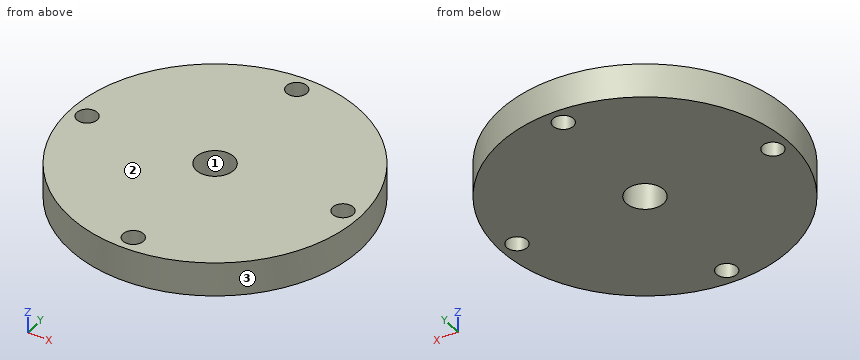
from build123d import *

# Parameters (mm, degrees)
ESQUISSE1_R        = 4.25
ESQUISSE1_R_2      = 0.3
ESQUISSE1_R_3      = 0.55
BOSS_EXTRU_1_DEPTH = 1


with BuildPart() as part:
    # Esquisse1 → Boss.-Extru.1 (new body)
    with BuildSketch(Plane.XY):
        Circle(ESQUISSE1_R)
        with Locations((0, 3.75)):
            Circle(ESQUISSE1_R_2, mode=Mode.SUBTRACT)
        Circle(ESQUISSE1_R_3, mode=Mode.SUBTRACT)
        with Locations((3.75, 0)):
            Circle(ESQUISSE1_R_2, mode=Mode.SUBTRACT)
        with Locations((0, -3.75)):
            Circle(ESQUISSE1_R_2, mode=Mode.SUBTRACT)
        with Locations((-3.75, 0)):
            Circle(ESQUISSE1_R_2, mode=Mode.SUBTRACT)
    extrude(amount=BOSS_EXTRU_1_DEPTH)


solid = part.part
For this review, take the finished solid that the model builds, in its own axes (mm). Face numbers are marked on the shaded views. Round coordinates to 2 decimals unless told otherwise and drop trailing zeros. Order: outer loops, then holes, each group sorted by start corner. A loop starts at its lowest first (then second) coordinate and runs counter-clockwise, first axis right, second up. Notation, with made-up numbers: (56.5, 20) -> (87.5, 20) arc R12 cw to (87.5, 27) -> close; hole circle Ø9 at (65.5, 49.5). An arc over 180 degrees is marked (long way). Put each result on its own line as item: value.
Q1. Mouldability with a two-part tool opening along X and no side actions: class the marked faces 1, 2 and 3 as pulls with the +X half, pulls with the -X half, needs draft (parallel to the pull), parting line crosses it, or undercut.
Check result:
face 1: undercut
face 2: needs draft
face 3: parting line crosses it
Q2. Add section B-B on y = -3.75. Write out the cut boundary in (x, z), plus the area to 3 significant figures.
Check result:
outline: (-2, 0) -> (-0.3, 0) -> (-0.3, 1) -> (-2, 1) -> close; (0.3, 0) -> (2, 0) -> (2, 1) -> (0.3, 1) -> close
area: 3.40 mm2
Q3. Add section C-C on z = 0.85. Write out the cut boundary in (x, y), plus the area to 3 significant figures.
Check result:
outline: circle Ø8.5 at (0, 0); hole circle Ø0.6 at (-3.75, 0); hole circle Ø1.1 at (0, 0); hole circle Ø0.6 at (0, -3.75); hole circle Ø0.6 at (0, 3.75); hole circle Ø0.6 at (3.75, 0)
area: 54.7 mm2
Q4. For probe 1 along Y at (x, z) = (0, 0.1); probe 2 along Y at (x, z) = (3.75, 0.3); probe 3 along Y at (x, z) = (1.5, 0.5), list the stretches that pass through material, from the lowest coordinate up. Write a range as [from, to].
Check result:
probe 1: [-4.25, -4.05], [-3.45, -0.55], [0.55, 3.45], [4.05, 4.25]
probe 2: [-2, -0.3], [0.3, 2]
probe 3: [-3.98, 3.98]
Q5. Add section A-A on x = 0. Write out the cut boundary in (y, z).
Check result:
outline: (-4.25, 0) -> (-4.05, 0) -> (-4.05, 1) -> (-4.25, 1) -> close; (-3.45, 0) -> (-0.55, 0) -> (-0.55, 1) -> (-3.45, 1) -> close; (0.55, 0) -> (3.45, 0) -> (3.45, 1) -> (0.55, 1) -> close; (4.05, 0) -> (4.25, 0) -> (4.25, 1) -> (4.05, 1) -> close
